Geometry check sheet. Reference: the model listing, model coordinates, mm. Round coordinates to 2 decimals unless told otherwise and drop trailing zeros. Write each loop counter-clockwise with the first axis right and the second up, starting at its lowest first coordinate (ties: lowest second). Pieces come first, ordered by that corner, then holes. Notation, with made-up numbers: M 72,60 L 92,60 A22 cw 92,83 Z; hole C 3.5,-34.5 d9. An arc over 180 degrees is marked long. Use a Markdown table: item, result.
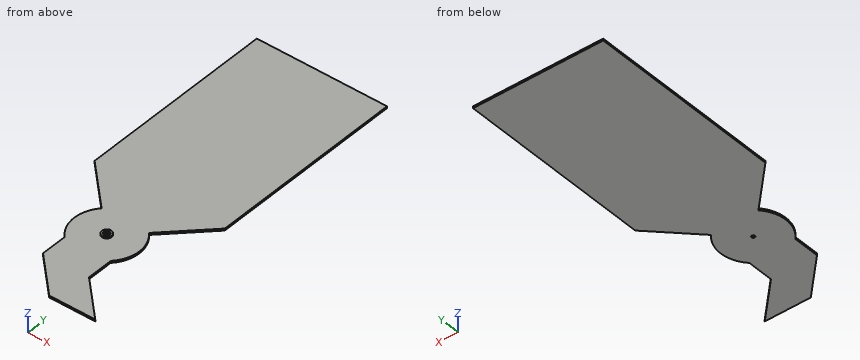
Autodesk Inventor part; units mm, degrees
ref_plane "YZ Plane" through (0, 0, 0) normal (1, 0, 0) x (0, 1, 0)
ref_plane "XZ Plane" through (0, 0, 0) normal (0, 1, 0) x (-1, 0, 0)
ref_plane "XY Plane" through (0, 0, 0) normal (0, 0, 1) x (1, 0, 0)
sketch "Sketch1" plane through (0, 0, 0) normal (0, 0, 1) x (1, 0, 0)
  line L0 (-100, 150) -> (100, 150)
  line L1 (100, 150) -> (100, -150)
  line L2 (-100, -150) -> (-100, 150)
  line L3 (-100, 150) -> (100, -150) construction
  line L4 (100, 150) -> (-100, -150) construction
  line L5 (100, -150) -> (36.4382, -213.5618)
  line L6 (-35.3571, -283.1536) -> (-35.3571, -323.1554)
  line L7 (-35.3571, -323.1554) -> (21.2114, -379.7239)
  line L8 (35.3571, -283.1536) -> (35.3571, -323.1554)
  line L9 (35.3571, -323.1554) -> (91.9257, -379.7239)
  line L10 (91.9257, -379.7239) -> (21.2114, -379.7239)
  arc A0 (-35.3571, -283.1536) -> (-35.3553, -283.1554) centre (0, -247.8) ccw
  arc A1 (-36.4382, -213.5618) -> (-35.3553, -283.1554) centre (0, -247.8) ccw
  arc A2 (35.3571, -283.1536) -> (36.4382, -213.5618) centre (0, -247.8) ccw
  line L11 (-100, -150) -> (-36.4382, -213.5618)
  point P0 (0, 0)
  point P1 (35.3571, -285.3571)
extrude "Extrusion1" add sketch "Sketch1" along normal blind 3
sketch "Sketch2" plane through (0, 0, 3) normal (0, 0, 1) x (1, 0, 0)
  arc A0 (35.3571, -283.1536) -> (36.4382, -213.5618) centre (0, -247.8) ccw
  circle A1 centre (0, -247.8) radius 2.5
  circle A2 centre (0, -247.8) radius 4.75
  circle A3 centre (0, -247.8) radius 7.5
  point P0 (0, 0)
  dimension "d20" = 5
  dimension "d21" = 9.5
  dimension "d22" = 15
extrude "Extrusion2" cut sketch "Sketch2" against normal blind 3 contours A1
extrude "Extrusion3" add sketch "Sketch2" along normal blind 2 contours A3
properties part number "leftside0"
Item 1: Cross-section at B-B, the plane x = 60.5. Record the cut outline in (y, z), and give its area (3 significant figures).
Outcome:
| item | result |
|---|---|
| outline | M -379.72,0 L -348.3,0 L -348.3,3 L -379.72,3 Z; M -189.5,0 L 150,0 L 150,3 L -189.5,3 Z |
| area | 1,110 mm2 |
Item 2: Cross-section at C-C, the plane x = -69. Record the cut outline in (y, z), and give its area (3 significant figures).
Outcome:
| item | result |
|---|---|
| outline | M -181,0 L 150,0 L 150,3 L -181,3 Z |
| area | 993 mm2 |
Item 3: Go/stop test with flat-tipped pins: pin 1 (4 mm diameter, centred on x = -52.5, y = -94.5, fed in from +Z); pin 2 (1.5 mm diameter, centred on y = -213.5, z = 1, fed in from -X); pin 3 (0.9 mm diameter, centred on y = -297, z = 1.5, fed in from +X); pin 4 (2 mm diameter, centred on x = -66, z = 4.5, fed in from -Y). Record where each tip stops, or that it passes through.
Outcome:
| item | result |
|---|---|
| pin 1 | stops at z = 3 |
| pin 2 | stops at x = -37.25 |
| pin 3 | stops at x = 35.36 |
| pin 4 | passes through |
Item 4: Cross-section at D-D, the plane y = -208. Record the cut outline in (x, z).
Outcome:
| item | result |
|---|---|
| outline | M -42,0 L 42,0 L 42,3 L -42,3 Z |
Item 5: Material ranges on line 1 along Y through (x, z) = (0, 3.8); line 2 along X through (y, z) = (-247.8, 0.7); line 3 along Z through (x, y) = (26, -51), recorded low to high. Write a range as from..to.
Outcome:
| item | result |
|---|---|
| line 1 | y = -255.3..-252.55, -243.05..-240.3 |
| line 2 | x = -50..-2.5, 2.5..50 |
| line 3 | z = 0..3 |
Item 6: Cross-section at A-A, the plane z = 1.3. Record the cut outline in (x, y).
Outcome:
| item | result |
|---|---|
| outline | M -100,-150 L -36.44,-213.56 A50 ccw -35.36,-283.15 L -35.36,-323.16 L 21.21,-379.72 L 91.93,-379.72 L 35.36,-323.16 L 35.36,-283.15 A50 ccw 36.44,-213.56 L 100,-150 L 100,150 L -100,150 Z; hole C 0,-247.8 d5 |
